For this review, take the finished solid that the model builds, in its own axes (mm). Face numbers are marked on the shaded views. A direction names the side the tool comes from. Coordinates: 2 decimals unless noted, no trailing zeros. Loops run counter-clockwise (first coordinate to the right, second up) from the corner with the lowest first, then second, coordinate; pieces in that order, holes last. Notation, with made-up numbers: M 20.5,32 L 36.5,32 A27 cw 36.5,59 Z; hole C 78.25,59.25 d1. An arc over 180 degrees is marked long. Answer as a JSON object with one key per item and string values. Group by question number.
Item 1: Add section D-D (y = -13). State the section outline as (x, z) points.
Item 2: Add section A-A (x = 0). State the section outline as (y, z) points.
Item 3: Wall thickness on L1, parallel to Z at x = -14.5, y = -4.5; L2, parallel to X at y = 6, z = -137.5; L3, parallel to X at y = 8.5, z = -41: over which ranges is each line inside the solid? List them lowest first. Write a range as from..to.
Item 4: Insertion check: pin 1 (1.5 mm diameter, centred on x = 3.5, y = -11, fed in from +Z); pin 2 (9 mm diameter, centred on y = 0.5, z = 33, fed in from +X); pin 3 (5 mm diameter, centred on y = -10, z = -102.5, fed in from +X). Each pin has a flat end and moves straight along its axis. Give the tip position at first contact, or say it passes through.
Item 5: Tool access review of the marked faces 1 and 2: name each direction out of +Z, -Z, +X, -X, +Y, -Y from which nothing blocks a thin tool from reaching the whole face with its end or side.
Item 6: Add section C-C (z = -104). State the section outline as (x, y) points, then the cut area to 3 significant figures.
Item 7: Add section B-B (y = 0). State the section outline as (x, z) points, then the cut area to 3 significant figures.
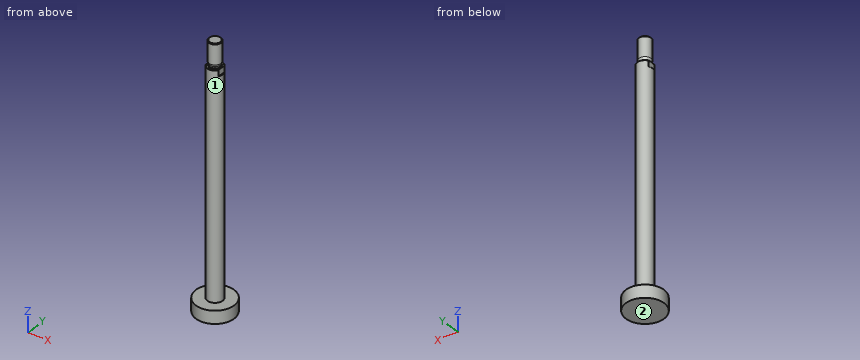
from build123d import *

# Parameters (mm, degrees)
CUT_EXTRUDE1_DEPTH      = 17
CUT_EXTRUDE1_DEPTH_BACK = 17


with BuildPart() as part:
    # Sketch1 → Revolve1 (revolve)
    with BuildSketch(Plane(origin=(0, 0, 0), x_dir=(0, 0, -1), z_dir=(1, 0, 0))):
        Polygon((-35.8, 0), (-35.8, 9.717157288), (-35.517157288, 10), (256.333333333, 10), (256.333333333, 25), (273, 25), (273, 0), align=None)
    revolve(axis=Axis((0, 0, -273), (0, 0, 1)))

    # Sketch2 → Cut-Extrude1 (cut, two sides)
    with BuildSketch(Plane(origin=(0, 0, 0), x_dir=(1, 0, 0), z_dir=(0, 1, 0))) as cut_extrude1_sk:
        Polygon((-17, -61.8), (17, -61.8), (17, -27.8), (8.5, -27.8), (8.5, -43.8), (-8.5, -43.8), (-8.5, -27.8), (-17, -27.8), align=None)
    extrude(amount=CUT_EXTRUDE1_DEPTH, mode=Mode.SUBTRACT)
    extrude(cut_extrude1_sk.sketch, amount=-CUT_EXTRUDE1_DEPTH_BACK, mode=Mode.SUBTRACT)

    # Sketch3 → Revolve2 (revolve)
    with BuildSketch(Plane(origin=(0, 0, 0), x_dir=(0, 0, -1), z_dir=(1, 0, 0))):
        with BuildLine():
            Line((-67.8, 0), (-67.8, 7.08))
            Line((-67.8, 7.08), (-66.88, 8))
            Line((-66.88, 8), (-41.28485129, 8))
            Line((-41.28485129, 8), (-38.524269872, 6.995230534))
            ThreePointArc((-38.524269872, 6.995230534), (-38.397990898, 6.961394185), (-38.267754764, 6.95))
            Line((-38.267754764, 6.95), (-36.55, 6.95))
            ThreePointArc((-36.55, 6.95), (-36.019669914, 7.169669914), (-35.8, 7.7))
            Line((-35.8, 7.7), (-35.05, 7.7))
            Line((-35.05, 7.7), (-35.05, 0))
            Line((-35.05, 0), (-67.8, 0))
        make_face()
    revolve(axis=Axis((0, 0, 35.05), (0, 0, 1)))


solid = part.part
From the geometry:
{
 "1": {"outline": "M -21.35,-273 L 21.35,-273 L 21.35,-256.33 L -21.35,-256.33 Z"},
 "2": {"outline": "M -25,-273 L 25,-273 L 25,-256.33 L 10,-256.33 L 10,35.52 L 9.72,35.8 L 7.7,35.8 A0.75 cw 6.95,36.55 L 6.95,38.27 A0.75 cw 7,38.52 L 8,41.28 L 8,66.88 L 7.08,67.8 L -7.08,67.8 L -8,66.88 L -8,41.28 L -7,38.52 A0.75 cw -6.95,38.27 L -6.95,36.55 A0.75 cw -7.7,35.8 L -9.72,35.8 L -10,35.52 L -10,-256.33 L -25,-256.33 Z"},
 "3": {"L1": "z = -273..-256.33", "L2": "x = -8..8", "L3": "x = -5.27..5.27"},
 "4": {"pin 1": "stops at z = -256.33", "pin 2": "stops at x = 8.5", "pin 3": "stops at x = 6.61"},
 "5": {"face 1": "+Z", "face 2": "-Z, +X, -X, +Y, -Y"},
 "6": {"outline": "C 0,0 d20", "area": "314 mm²"},
 "7": {"outline": "M -25,-273 L 25,-273 L 25,-256.33 L 10,-256.33 L 10,27.8 L 8.5,27.8 L 8.5,35.8 L 7.7,35.8 A0.75 cw 6.95,36.55 L 6.95,38.27 A0.75 cw 7,38.52 L 8,41.28 L 8,66.88 L 7.08,67.8 L -7.08,67.8 L -8,66.88 L -8,41.28 L -7,38.52 A0.75 cw -6.95,38.27 L -6.95,36.55 A0.75 cw -7.7,35.8 L -8.5,35.8 L -8.5,27.8 L -10,27.8 L -10,-256.33 L -25,-256.33 Z", "area": "7,150 mm²"}
}
